from build123d import *

# Parameters (mm, degrees)
IZIM1_R               = 4.825
BOSS_EXTRUDE1_DEPTH   = 15
IZIM1_6_R             = 2.5
CUT_EXTRUDE1_DEPTH    = 3
SKETCH2_R             = 2.5
CUT_EXTRUDE2_DEPTH    = 5
SKETCH3_R             = 1
CUT_EXTRUDE3_DEPTH    = 5.825
IZIM2_W               = 4
IZIM2_H               = 1.5
KES_EKSTR_ZYON1_DEPTH = 4


with BuildPart() as part:
    # Çizim1 → Boss-Extrude1 (new body)
    with BuildSketch(Plane(origin=(0, 0, 0), x_dir=(1, 0, 0), z_dir=(0, 1, 0))):
        Circle(IZIM1_R)
    extrude(amount=BOSS_EXTRUDE1_DEPTH)

    # Çizim1<6> → Cut-Extrude1 (cut)
    with BuildSketch(Plane(origin=(0, 0, 0), x_dir=(1, 0, 0), z_dir=(0, 1, 0))):
        Circle(IZIM1_6_R)
    extrude(amount=CUT_EXTRUDE1_DEPTH, mode=Mode.SUBTRACT)

    # Sketch2 → Cut-Extrude2 (cut)
    with BuildSketch(Plane(origin=(0, 15, 0), x_dir=(1, 0, 0), z_dir=(0, 1, 0))):
        Circle(SKETCH2_R)
    extrude(amount=-CUT_EXTRUDE2_DEPTH, mode=Mode.SUBTRACT)

    # Sketch3 → Cut-Extrude3 (cut, through all)
    with BuildSketch(Plane.XY):
        with Locations((0, 13)):
            Circle(SKETCH3_R)
    extrude(amount=-CUT_EXTRUDE3_DEPTH, mode=Mode.SUBTRACT)

    # Çizim2 → Kes-Ekstrüzyon1 (cut)
    with BuildSketch(Plane(origin=(0, 15, 0), x_dir=(1, 0, 0), z_dir=(0, 1, 0))):
        with Locations((0, 3.45)):
            Rectangle(IZIM2_W, IZIM2_H)
    extrude(amount=-KES_EKSTR_ZYON1_DEPTH, mode=Mode.SUBTRACT)


solid = part.part
The listing builds one solid part. Answer for the finished solid, in the listing's coordinates (mm). A direction names the side the tool comes from. Round coordinates to 2 decimals unless told otherwise and drop trailing zeros. Loops run counter-clockwise (first coordinate to the right, second up) from the corner with the lowest first, then second, coordinate; pieces in that order, holes last. Notation, with made-up numbers: M -19.75,21.25 L 26.25,21.25 A26 ccw 26.25,59.25 Z; hole C 65.5,7.25 d4. An arc over 180 degrees is marked long. Return JSON: item names as keys, results as strings.
Q1. Find section B-B, the plane z = 0. Determine the outline of the cut face in (x, y) (3 decimals).
Results list:
{"outline": "M -4.825,0 L -2.5,0 L -2.5,3 L 2.5,3 L 2.5,0 L 4.825,0 L 4.825,15 L 2.5,15 L 2.5,10 L -2.5,10 L -2.5,15 L -4.825,15 Z"}
Q2. Find section D-D, the plane y = 12.25. Determine the outline of the cut face in (x, z) (3 decimals), plus the area to 3 significant figures.
Results list:
{"outline": "M -2,-4.2 L -2,-2.7 L -0.661,-2.7 L -0.661,-2.411 A2.5 cw long 0.661,-2.411 L 0.661,-2.7 L 2,-2.7 L 2,-4.2 L 0.661,-4.2 L 0.661,-4.779 A4.825 ccw long -0.661,-4.779 L -0.661,-4.2 Z", "area": "46.4 mm2"}
Q3. Which of the six approach directions +Z, -Z, +X, -X, +Y, -Y give full straight-line access (tool end or side, diameter ignored) to faces 4 (the face through (0.954, 13.3, -2.538)), 5 (the face through (-0.54, 1.48, 2.44)), 6 (the face through (2, 15, 2)), 7 (the face through (0, 11, -3))?
Results list:
{"face 4": "-Z", "face 5": "-Y", "face 6": "+Z, -Z, +X, -X, +Y", "face 7": "+Y"}
Q4. The mould has two halves that part along X. Classify faces 1 (the face through (-1, 14, -4.2)), 2 (the face through (2, 0, 2)), 3 (the face through (-1.05, 7.4, 4.71)): released by +X, released by -X, zero draft, split by the parting line, or undercut.
Results list:
{"face 1": "undercut", "face 2": "zero draft", "face 3": "split by the parting line"}
Q5. Each of these flat-tipped pins is pushed along its axis until it touches: pin 1 Ø1.2 at (x, y) = (0.5, 12.5) entering from -Z; pin 2 Ø0.8 at (y, z) = (13, -4) entering from -X; pin 3 Ø1 at (y, z) = (12, -1.5) entering from -X. Where does it stop, or does it pass through?
Results list:
{"pin 1": "stops at z = -4.82", "pin 2": "stops at x = -3.21", "pin 3": "stops at x = -4.72"}
Q6. Find the intervals of material crossed by line 1 along Y through (x, z) = (0, -4.6); line 2 along Y through (x, z) = (-0.5, -3); line 3 along X through (y, z) = (13, -4.3), in increasing order. Write a range as from..to.
Results list:
{"line 1": "y = 0..12, 14..15", "line 2": "y = 0..11", "line 3": "x = -2.19..-1, 1..2.19"}
Q7. Find section A-A, the plane x = 0. Determine the outline of the cut face in (y, z) (3 decimals).
Results list:
{"outline": "M 0,-4.825 L 12,-4.825 L 12,-4.2 L 11,-4.2 L 11,-2.7 L 12,-2.7 L 12,-2.5 L 10,-2.5 L 10,2.5 L 15,2.5 L 15,4.825 L 0,4.825 L 0,2.5 L 3,2.5 L 3,-2.5 L 0,-2.5 Z; M 14,-4.825 L 15,-4.825 L 15,-4.2 L 14,-4.2 Z; M 14,-2.7 L 15,-2.7 L 15,-2.5 L 14,-2.5 Z"}
Q8. Find section C-C, the plane y = 10.5. Determine the outline of the cut face in (x, z) (3 decimals), plus the area to 3 significant figures.
Results list:
{"outline": "C 0,0 d9.65; hole C 0,0 d5", "area": "53.5 mm2"}
